The listing builds one solid part. Answer for the finished solid, in the listing's coordinates (mm). A direction names the side the tool comes from. Give positions to 0.01 mm unless a question says otherwise; leave off trailing zeros. Write each loop counter-clockwise with the first axis right and the second up, starting at its lowest first coordinate (ties: lowest second). Pieces come first, ordered by that corner, then holes. Notation, with made-up numbers: (64, 30) - (123, 30) arc R22 cw to (123, 50) - close; hole circle Ø6 at (66, 83). An arc over 180 degrees is marked (long way). One line per question, with ' | ' between items. Start each with the question number.
1. The mould has two halves that part along Z. Classify faces 1 (the face through (8, 0, 38)), 2 (the face through (-41.5, -0.14, 58.64)), 3 (the face through (-98, 0, 80)), 4 (the face through (39.765, -0.14, 20.396)): +Z half, -Z half, draft (parallel to the pull), parting line (faces both ways), or undercut.
2. A cutting plane is placed at B-B (y = 0). Determine the outline of the cut face in (x, z).
3. Given P1, Ø5, axis at x = -28.5, z = 58.5, coming from the -Y side; P2, Ø5, axis at x = 23.5, y = 4.5, coming from the +Z side; P3, Ø10, axis at x = -97, y = 3.5, coming from the -Z side; P4, Ø1, axis at y = -0.5, z = 64, coming from the -X side, each flat-ended and moving along its own axis, determine where each tip first touches the part or whether it passes through.
4. For faces 5 (the face through (-90, 0, 78)), 6 (the face through (-15.288, -0.14, 39.565)), 7 (the face through (8, 0, 42)), determine the directions among +Z, -Z, +X, -X, +Y, -Y from which every point of the face is accessible in a straight line to the end or side of a thin tool.
5. A cutting plane is placed at C-C (x = 0). Determine the outline of the cut face in (y, z).
6. A cutting plane is placed at D-D (z = 40). Determine the outline of the cut face in (x, y).
7. A cutting plane is placed at A-A (x = -95). Determine the outline of the cut face in (y, z), then the cut area to 3 significant figures.
8. Find the intervals of material crossed by L1, parallel to Z at x = 0.5, y = 5; L2, parallel to Y at x = 0, z = -1; L3, parallel to Z at x = 35, y = -8.75, in increasing order. Write a range as from..to.
```python
from build123d import *

# Parameters (mm, degrees)
F1_DEPTH = 10
F2_R     = 3
F3_DEPTH = 50
F4_R     = 3
F5_DEPTH = 25


with BuildPart() as f1:
    # F0 (on Front) → F1 (new body, symmetric)
    with BuildSketch(Plane.XZ):
        with BuildLine():
            ThreePointArc((-56.90276, 76.083458), (-64.832339, 80.477965), (-73.769526, 82))
            Line((-73.769526, 82), (-105, 82))
            ThreePointArc((-105, 82), (-107, 80), (-105, 78))
            Line((-105, 78), (-73.769526, 78))
            ThreePointArc((-73.769526, 78), (-66.156367, 76.703451), (-59.40154, 72.959983))
            Line((-59.40154, 72.959983), (-23.09724, 43.916542))
            ThreePointArc((-23.09724, 43.916542), (-15.167661, 39.522035), (-6.230474, 38))
            Line((-6.230474, 38), (1.769526, 38))
            Line((1.769526, 38), (21.769526, 38))
            ThreePointArc((21.769526, 38), (39.769526, 20), (21.769526, 2))
            Line((21.769526, 2), (1.769526, 2))
            Line((1.769526, 2), (-8.230474, 2))
            ThreePointArc((-8.230474, 2), (-10.230474, 0), (-8.230474, -2))
            Line((-8.230474, -2), (1.769526, -2))
            Line((1.769526, -2), (21.769526, -2))
            ThreePointArc((21.769526, -2), (43.769526, 20), (21.769526, 42))
            Line((21.769526, 42), (1.769526, 42))
            Line((1.769526, 42), (-6.230474, 42))
            ThreePointArc((-6.230474, 42), (-13.843633, 43.296549), (-20.59846, 47.040017))
            Line((-20.59846, 47.040017), (-56.90276, 76.083458))
        make_face()
    extrude(amount=F1_DEPTH, both=True)

    # F2 (on Top) → F3 (cut, symmetric)
    with BuildSketch(Plane.XY):
        Circle(F2_R)
    extrude(amount=F3_DEPTH, both=True, mode=Mode.SUBTRACT)

    # F4 (on face) → F5 (cut)
    with BuildSketch(Plane.XY.offset(82)):
        with Locations((-95, 0)):
            Circle(F4_R)
    extrude(amount=-F5_DEPTH, mode=Mode.SUBTRACT)


solid = f1.part
```
Determined:
1) face 1: undercut | face 2: -Z half | face 3: draft | face 4: undercut
2) outline: (-105, 78) - (-98, 78) - (-98, 82) - (-105, 82) arc R2 ccw to start; (-92, 78) - (-73.77, 78) arc R23 cw to (-59.4, 72.96) - (-23.1, 43.92) arc R27 ccw to (-6.23, 38) - (-3, 38) - (-3, 42) - (-6.23, 42) arc R23 cw to (-20.6, 47.04) - (-56.9, 76.08) arc R27 ccw to (-73.77, 82) - (-92, 82) - close; (-8.23, -2) - (-3, -2) - (-3, 2) - (-8.23, 2) arc R2 ccw to start; (3, -2) - (21.77, -2) arc R22 ccw to (21.77, 42) - (3, 42) - (3, 38) - (21.77, 38) arc R18 cw to (21.77, 2) - (3, 2) - close
3) P1: through | P2: z = 42 | P3: z = 78 | P4: x = -48.83
4) face 5: -Z, -X, +Y, -Y | face 6: -X, +Y, -Y | face 7: +Z, +X, +Y, -Y
5) outline: (-10, -2) - (-3, -2) - (-3, 2) - (-10, 2) - close; (-10, 38) - (-3, 38) - (-3, 42) - (-10, 42) - close; (3, -2) - (10, -2) - (10, 2) - (3, 2) - close; (3, 38) - (10, 38) - (10, 42) - (3, 42) - close
6) outline: (-16.43, -10) - (30.93, -10) - (30.93, 10) - (-16.43, 10) - close; hole circle Ø6 at (0, 0)
7) outline: (-10, 78) - (-3, 78) - (-3, 82) - (-10, 82) - close; (3, 78) - (10, 78) - (10, 82) - (3, 82) - close | area: 56.0 mm2
8) L1: -2..2, 38..42 | L2: -10..-3, 3..10 | L3: 2.42..7.8, 32.2..37.58
